```python
from build123d import *

# Parameters (mm, degrees)
SKETCH_2_W          = 30
SKETCH_2_H          = 12
SKETCH_2_R          = 2
EXTRUDE_1_DEPTH     = 1
SKETCH_3_R          = 3.2
SKETCH_3_R_2        = 2
EXTRUDE_2_DEPTH     = 1.7
SKETCH_4_R          = 1
CUT_EXTRUDE_1_DEPTH = 5
EXTRUDE_3_DEPTH     = 12
SKETCH_6_W          = 2
SKETCH_6_H          = 12
CUT_EXTRUDE_2_DEPTH = 1


with BuildPart() as part:
    # 草图2 → 凸台-拉伸1 (new body)
    with BuildSketch(Plane(origin=(0, 0, 0), x_dir=(1, 0, 0), z_dir=(0, 1, 0))):
        with Locations((-3.527606217, -1.94741871)):
            Rectangle(SKETCH_2_W, SKETCH_2_H)
        with Locations(Location((-5.207606217, -1.94741871, 0), (0, 0, 270))):
            Circle(SKETCH_2_R, mode=Mode.SUBTRACT)
    extrude(amount=EXTRUDE_1_DEPTH)

    # 草图3 → 凸台-拉伸2 (add)
    with BuildSketch(Plane(origin=(0, 1, 0), x_dir=(1, 0, 0), z_dir=(0, 1, 0))):
        with Locations(Location((-5.207606217, -1.94741871, 0), (0, 0, 270))):
            Circle(SKETCH_3_R)
        with Locations(Location((-5.207606217, -1.94741871, 0), (0, 0, 270))):
            Circle(SKETCH_3_R_2, mode=Mode.SUBTRACT)
    extrude(amount=EXTRUDE_2_DEPTH)

    # 草图4 → 切除-拉伸1 (cut)
    with BuildSketch(Plane.XZ):
        with Locations(Location((-10.481209657, -0.12271673, 0), (0, 0, 270))):
            Circle(SKETCH_4_R)
    extrude(amount=-CUT_EXTRUDE_1_DEPTH, mode=Mode.SUBTRACT)

    # 草图5 → 凸台-拉伸3 (add)
    with BuildSketch(Plane(origin=(0, 0, -4.05258129), x_dir=(-1, 0, 0), z_dir=(0, 0, -1))):
        Polygon((18.527606217, 1), (18.527606217, 0), (19.527606217, 1), align=None)
    extrude(amount=-EXTRUDE_3_DEPTH)

    # 草图6 → 切除-拉伸2 (cut)
    with BuildSketch(Plane.XZ):
        with Locations((10.472393783, 1.94741871)):
            Rectangle(SKETCH_6_W, SKETCH_6_H)
    extrude(amount=-CUT_EXTRUDE_2_DEPTH, mode=Mode.SUBTRACT)


solid = part.part
```
Geometry check sheet. Reference: the model listing, model coordinates, mm. A direction names the side the tool comes from. Round coordinates to 2 decimals unless told otherwise and drop trailing zeros. Loops run counter-clockwise (first coordinate to the right, second up) from the corner with the lowest first, then second, coordinate; pieces in that order, holes last. Notation, with made-up numbers: (24, -27) - (69, -27) arc R21 cw to (69, -23) - close; hole circle Ø10 at (3.25, 11). An arc over 180 degrees is marked (long way). Write each question's results on one line, items separated by ' | '. Start each with the question number.
Q1. Cross-section at D-D on x = -13.25. Enter the section's corners in (y, z).
Q2. Thickness scan on line 1 (X direction, y = 2.45, z = 2); line 2 (Y direction, x = -18.25, z = -1.25); line 3 (X direction, y = 1.75, z = 0.5). Record the ranges inside material, lowest first. Write a range as [from, to].
Q3. Access from +Z, -Z, +X, -X, +Y, -Y to the whole of each face (thin tool, end or side, straight path). Record for faces 4 (the cylindrical face through (-2.035, 1.838, 1.531)), 5 (the flat face through (-4.8, 0.5, -4.053)).
Q4. Cross-section at A-A on x = -5.75. Enter the section's corners in (y, z), and give its area (3 significant figures).
Q5. Cross-section at C-C on z = 4.75. Enter the section's corners in (x, y).
Q6. Release check for a two-part mould opening along Z. For faces 1 (the cylindrical face through (-6.98, 1.33, 2.87)), 2 (the flat face through (-4.8, 0.5, 7.947)), 3 (the flat face through (9.472, 0.5, 1.9)) record: +Z half, -Z half, draft (parallel to the pull), parting line (faces both ways), or undercut.
Q7. Cross-section at B-B on z = -0.5. Enter the section's corners in (x, y), and give its area (3 significant figures).
Q8. Gauge pin test, flat ends, axial feed: P1, Ø2.5, axis at x = -5.21, z = 1.95, coming from the -Y side; P2, Ø3.5, axis at x = -11, z = 3.5, coming from the +Y side. Record the tip position at first contact, or that the pin passes through.
Answers below:
1) outline: (0, -4.05) - (1, -4.05) - (1, 7.95) - (0, 7.95) - close
2) line 1: x = [-8.41, -7.21], [-3.21, -2.01] | line 2: y = [0, 1] | line 3: x = [-8.06, -6.59], [-3.83, -2.35]
3) face 4: +Y | face 5: -Z, +X, -X, +Y, -Y
4) outline: (0, -4.05) - (1, -4.05) - (1, -1.21) - (2.7, -1.21) - (2.7, 0.02) - (0, 0.02) - close; (0, 3.87) - (2.7, 3.87) - (2.7, 5.1) - (1, 5.1) - (1, 7.95) - (0, 7.95) - close | area: 12.3 mm²
5) outline: (-19.53, 1) - (-18.53, 0) - (9.47, 0) - (9.47, 1) - (-3.66, 1) - (-3.66, 2.7) - (-6.75, 2.7) - (-6.75, 1) - close
6) face 1: undercut | face 2: +Z half | face 3: draft
7) outline: (-19.53, 1) - (-18.53, 0) - (-11.41, 0) - (-11.41, 1) - close; (-9.56, 0) - (9.47, 0) - (9.47, 1) - (-3.15, 1) - (-3.15, 2.7) - (-7.27, 2.7) - (-7.27, 1) - (-9.56, 1) - close | area: 33.7 mm²
8) P1: passes through | P2: stops at y = 1
